Part print with two shaded views. Sizes in mm from the minimum x, y, z corner. A direction names the side the tool comes from. Round coordinates to 2 decimals unless told otherwise and drop trailing zeros. Order: outer loops, then holes, each group sorted by start corner. A loop starts at its lowest first (then second) coordinate and runs counter-clockwise, first axis right, second up. Notation, with made-up numbers: M -23,-13.5 L -9,-13.5 A20 cw -9,-8.5 Z; hole C 87,34.5 d4. An arc over 180 degrees is marked long. Answer as a JSON object with one key per item and string values.
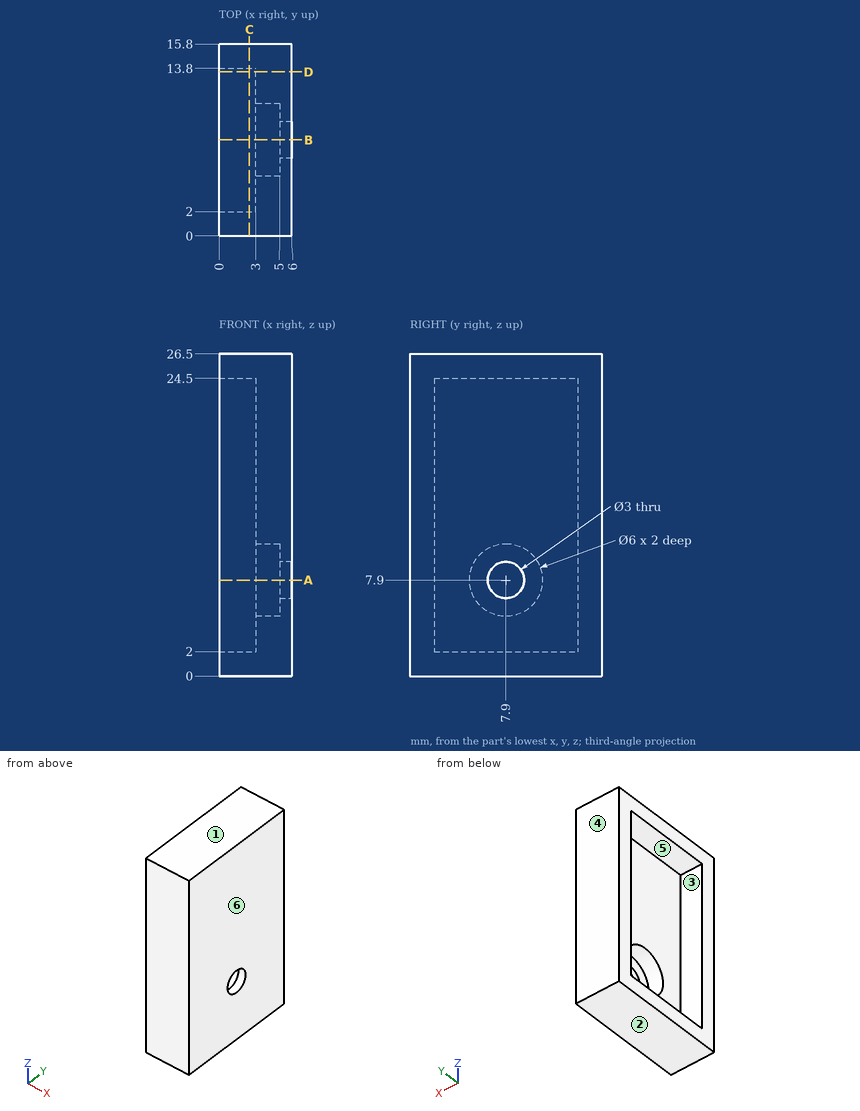
Item 1: Saw through at C-C on x = 2.5. List the corners of the cut face in (y, z).
Worked answers:
{"outline": "M 0,0 L 15.8,0 L 15.8,26.5 L 0,26.5 Z; hole M 2,2 L 13.8,2 L 13.8,24.5 L 2,24.5 Z"}
Item 2: Drop flat-ended pins along their axis: pin 1 Ø5 at (y, z) = (8, 9) entering from -X; pin 2 Ø5 at (y, z) = (7.9, 7.9) entering from -X. Give the stop position or say it passes through.
Worked answers:
{"pin 1": "stops at x = 3", "pin 2": "stops at x = 5"}
Item 3: 3-axis set-ups, long thin cutter, end or side, ignore diameter. For the marked faces 5 and 6: which of +Z, -Z, +X, -X, +Y, -Y reach the whole face in a straight line?
Worked answers:
{"face 5": "-X", "face 6": "+Z, -Z, +X, +Y, -Y"}
Item 4: Saw through at B-B on y = 7.9. List the corners of the cut face in (x, z), and give its area (3 significant figures).
Worked answers:
{"outline": "M 0,0 L 6,0 L 6,6.4 L 5,6.4 L 5,4.9 L 3,4.9 L 3,2 L 0,2 Z; M 0,24.5 L 3,24.5 L 3,10.9 L 5,10.9 L 5,9.4 L 6,9.4 L 6,26.5 L 0,26.5 Z", "area": "76.5 mm2"}
Item 5: Two-plate mould, pull along Z, no slides. Class the marked faces 1, 2, 3 and 4: released by +Z, released by -Z, zero draft, split by the parting line, or undercut.
Worked answers:
{"face 1": "released by +Z", "face 2": "released by -Z", "face 3": "undercut", "face 4": "zero draft"}
Item 6: Saw through at D-D on y = 13.5. List the corners of the cut face in (x, z).
Worked answers:
{"outline": "M 0,0 L 6,0 L 6,26.5 L 0,26.5 L 0,24.5 L 3,24.5 L 3,2 L 0,2 Z"}
Item 7: Wall check: line 1 along Y through (x, z) = (1.5, 17.25); line 2 along Y through (x, z) = (4.1, 7.9); line 3 along Z through (x, y) = (5.4, 7.9). Give the ranges that are in metal, low to high. Write a range as [from, to].
Worked answers:
{"line 1": "y = [0, 2], [13.8, 15.8]", "line 2": "y = [0, 4.9], [10.9, 15.8]", "line 3": "z = [0, 6.4], [9.4, 26.5]"}
Item 8: Saw through at A-A on z = 7.9. List the corners of the cut face in (x, y).
Worked answers:
{"outline": "M 0,0 L 6,0 L 6,6.4 L 5,6.4 L 5,4.9 L 3,4.9 L 3,2 L 0,2 Z; M 0,13.8 L 3,13.8 L 3,10.9 L 5,10.9 L 5,9.4 L 6,9.4 L 6,15.8 L 0,15.8 Z"}
